Job drawing, mm, ordinate dimensions from the low corner. One solid piece. A direction names the side the tool comes from. Coordinates: 2 decimals unless noted, no trailing zeros. Write each loop counter-clockwise with the first axis right and the second up, starting at its lowest first coordinate (ties: lowest second). Pieces come first, ordered by that corner, then holes. Notation, with made-up numbers: (9.5, 57) - (36.5, 57) arc R30 cw to (36.5, 94) - close; hole circle Ø10 at (-28, 63). An arc over 180 degrees is marked (long way). Use a Markdown table: item, result.
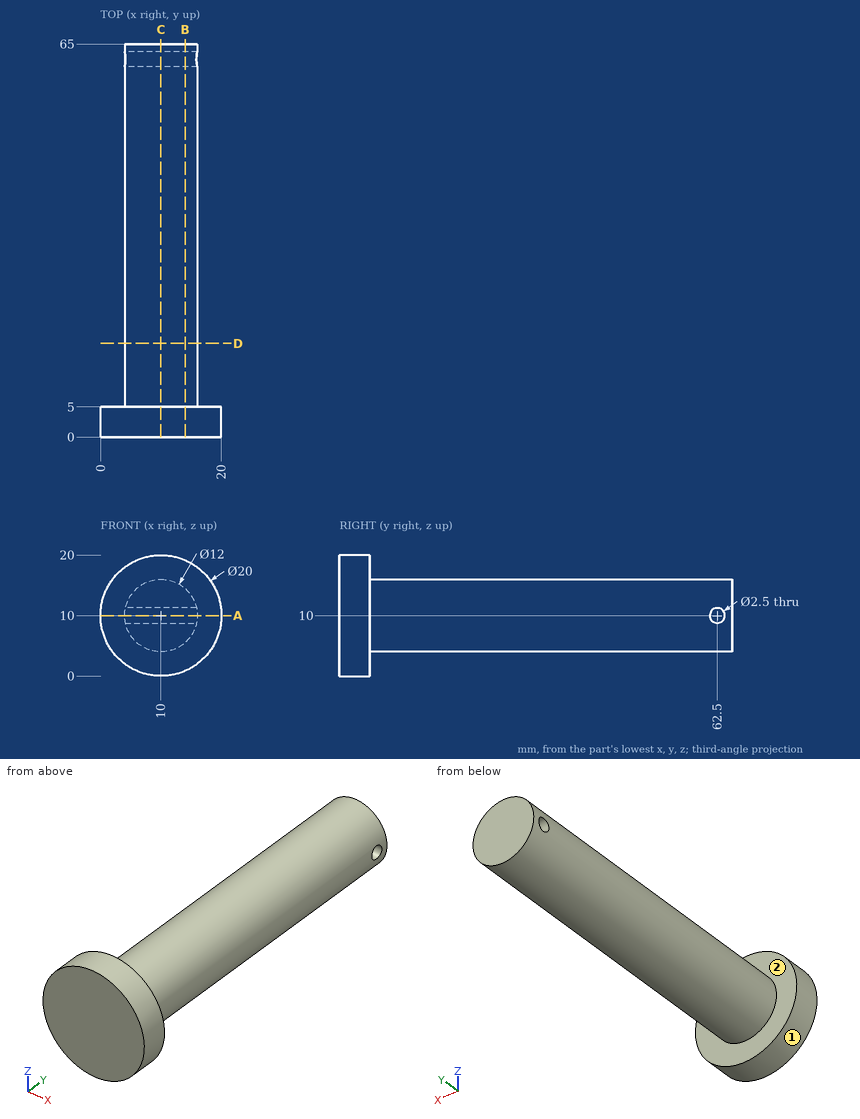
Item 1: Band-saw the part on A-A, the plane z = 10. Give the cut face in (x, y), then the cut area to 3 significant figures.
From the geometry:
| item | result |
|---|---|
| outline | (0, 0) - (20, 0) - (20, 5) - (16, 5) - (16, 61.25) - (4, 61.25) - (4, 5) - (0, 5) - close; (4, 63.75) - (16, 63.75) - (16, 65) - (4, 65) - close |
| area | 790 mm^2 |
Item 2: Band-saw the part on B-B, the plane x = 14. Give the cut face in (y, z).
From the geometry:
| item | result |
|---|---|
| outline | (0, 0.83) - (5, 0.83) - (5, 5.53) - (65, 5.53) - (65, 14.47) - (5, 14.47) - (5, 19.17) - (0, 19.17) - close; hole circle Ø2.5 at (62.5, 10) |
Item 3: Which spindle directions (+Z, -Z, +X, -X, +Y, -Y) get a long thin tool onto all of the face, cutting with end or side? Do the marked faces 1 and 2. Say none if no direction does.
From the geometry:
| item | result |
|---|---|
| face 1 | +Y, -Y |
| face 2 | +Y |
Item 4: Drill centre lines: probe 1 along Y at (x, z) = (13, 10); probe 2 along Y at (x, z) = (10.5, 17.75); probe 3 along Z at (x, y) = (9.75, 62.5). Where is each one in solid material? Low to high.
From the geometry:
| item | result |
|---|---|
| probe 1 | 0 to 61.25, 63.75 to 65 |
| probe 2 | 0 to 5 |
| probe 3 | 4.01 to 8.75, 11.25 to 15.99 |
Item 5: Band-saw the part on D-D, the plane y = 15.5. Give the cut face in (x, z).
From the geometry:
| item | result |
|---|---|
| outline | circle Ø12 at (10, 10) |
Item 6: Drop flat-ended pins along their axis: P1, Ø6, axis at y = 38, z = 5, coming from the -X side; P2, Ø4, axis at x = 7.5, y = 7.5, coming from the +Z side; P3, Ø3, axis at y = 39, z = 9, coming from the -X side. Give the stop position or say it passes through.
From the geometry:
| item | result |
|---|---|
| P1 | x = 4.34 |
| P2 | z = 15.98 |
| P3 | x = 4 |
Item 7: Band-saw the part on C-C, the plane x = 10. Give the cut face in (y, z), then the cut area to 3 significant figures.
From the geometry:
| item | result |
|---|---|
| outline | (0, 0) - (5, 0) - (5, 4) - (65, 4) - (65, 16) - (5, 16) - (5, 20) - (0, 20) - close; hole circle Ø2.5 at (62.5, 10) |
| area | 815 mm^2 |
